from build123d import *
from build123d.topology import SkipClean

# Parameters (mm, degrees)
SKETCH1_R           = 75
SKETCH1_R_2         = 73
BOSS_EXTRUDE1_DEPTH = 25
BOSS_EXTRUDE2_START = -25
BOSS_EXTRUDE2_DEPTH = 25
SKETCH4_R           = 12
CUT_EXTRUDE2_DEPTH  = 81
BOSS_EXTRUDE3_START = 2
SKETCH5_R           = 75
SKETCH5_R_2         = 12
BOSS_EXTRUDE3_DEPTH = 2
CHAMFER1_SIZE       = 2
SKETCH6_R           = 14
SKETCH6_R_2         = 12
BOSS_EXTRUDE4_DEPTH = 50
SKETCH7_R           = 16
SKETCH7_R_2         = 14
BOSS_EXTRUDE5_DEPTH = 3
BOSS_EXTRUDE6_START = -2
SKETCH8_R           = 78
SKETCH8_R_2         = 75
BOSS_EXTRUDE6_DEPTH = 2


with BuildPart() as part:
    # Sketch1 → Boss-Extrude1 (new body)
    with BuildSketch(Plane.XY):
        Circle(SKETCH1_R)
        Circle(SKETCH1_R_2, mode=Mode.SUBTRACT)
    extrude(amount=BOSS_EXTRUDE1_DEPTH)

    # Sketch2 → Boss-Extrude2 (add)
    with BuildSketch(Plane.XY.offset(25).offset(BOSS_EXTRUDE2_START)):
        with BuildLine():
            Line((75, 81.287132565), (48, 81.287132565))
            Line((48, 81.287132565), (48, 57.628118137))
            ThreePointArc((48, 57.628118137), (67.915388536, 31.819805153), (75, 0))
            Line((75, 0), (75, 81.287132565))
        make_face()
    extrude(amount=BOSS_EXTRUDE2_DEPTH)

    # Sketch4 → Cut-Extrude2 (cut)
    with BuildSketch(Plane(origin=(0, 81.287132565, 0), x_dir=(1, 0, 0), z_dir=(0, 1, 0))):
        with Locations(Location((61.5, -12.5, 0), (0, 0, 270))):
            Circle(SKETCH4_R)
    extrude(amount=-CUT_EXTRUDE2_DEPTH, mode=Mode.SUBTRACT)

    # Sketch5 → Boss-Extrude3 (add)
    with BuildSketch(Plane(origin=(0, 0, 0), x_dir=(-1, 0, 0), z_dir=(0, 0, -1)).offset(BOSS_EXTRUDE3_START)):
        Circle(SKETCH5_R)
        Circle(SKETCH5_R_2, mode=Mode.SUBTRACT)
    extrude(amount=-BOSS_EXTRUDE3_DEPTH)

    # Chamfer1
    # the kernel refuses this chamfer: 2 mm, written as the material it takes off along each edge
    with BuildSketch(Plane(origin=(75, 81.287132565, -5.143365976), x_dir=(0.027495876610589005, -0.9996219169112968, 0), z_dir=(0, 0, 1))) as chamfer1_piece_1:
        Polygon((CHAMFER1_SIZE * 0.999621916911, -CHAMFER1_SIZE * 0.0274958766106), (-CHAMFER1_SIZE * 0.0274958766106, -CHAMFER1_SIZE * 0.999621916911), (0, 0), align=None)
    extrude(amount=35.286731952, mode=Mode.SUBTRACT)
    with BuildSketch(Plane(origin=(48, 81.287132565, -5.143365976), x_dir=(-0.02749587661058555, -0.9996219169112968, 0), z_dir=(0, 0, 1))) as chamfer1_piece_2:
        Polygon((CHAMFER1_SIZE * 0.999621916911, CHAMFER1_SIZE * 0.0274958766106), (-CHAMFER1_SIZE * 0.0274958766106, CHAMFER1_SIZE * 0.999621916911), (0, 0), align=None)
    extrude(amount=35.286731952, mode=Mode.SUBTRACT)
    with BuildSketch(Plane(origin=(80.143365976, 81.287132565, 25), x_dir=(0, -0.9996219169112968, 0.02749587661058555), z_dir=(-1, 0, 0)), Plane(origin=(80.143365976, 81.287132565, 0), x_dir=(0, 0.02749587661058908, 0.9996219169112968), z_dir=(-1, 0, 0))) as chamfer1_piece_3:
        Polygon((CHAMFER1_SIZE * 0.999621916911, -CHAMFER1_SIZE * 0.0274958766106), (-CHAMFER1_SIZE * 0.0274958766106, -CHAMFER1_SIZE * 0.999621916911), (0, 0), align=None)
    extrude(amount=37.286731952, mode=Mode.SUBTRACT)

    # Sketch6 → Boss-Extrude4 (add)
    with SkipClean():  # the faces are left unmerged after this step: merging them gives an invalid solid
        with BuildSketch(Plane.XY):
            with Locations(Location((0, 0, 0), (0, 0, 180))):
                Circle(SKETCH6_R)
            Circle(SKETCH6_R_2, mode=Mode.SUBTRACT)
        extrude(amount=BOSS_EXTRUDE4_DEPTH)
    add(part.part.scale(1), mode=Mode.REPLACE)  # the faces are merged on a copy

    # Sketch7 → Boss-Extrude5 (add)
    with BuildSketch(Plane.XY):
        with Locations(Location((0, 0, 0), (0, 0, 180))):
            Circle(SKETCH7_R)
        Circle(SKETCH7_R_2, mode=Mode.SUBTRACT)
    extrude(amount=BOSS_EXTRUDE5_DEPTH)

    # Sketch8 → Boss-Extrude6 (add)
    with SkipClean():  # the faces are left unmerged after this step: merging them gives an invalid solid
        with BuildSketch(Plane.XY.offset(25).offset(BOSS_EXTRUDE6_START)):
            Circle(SKETCH8_R)
            with Locations(Location((0, 0, 0), (0, 0, 180))):
                Circle(SKETCH8_R_2, mode=Mode.SUBTRACT)
        extrude(amount=BOSS_EXTRUDE6_DEPTH)


solid = part.part
Read the model definition and answer for the solid it produces. Units are mm, in the model's axes. A direction names the side the tool comes from. Coordinates: 2 decimals unless noted, no trailing zeros. Loops run counter-clockwise (first coordinate to the right, second up) from the corner with the lowest first, then second, coordinate; pieces in that order, holes last. Notation, with made-up numbers: (78, -11) -> (106, -11) arc R31 cw to (106, 27) -> close; hole circle Ø1 at (64, 62). An arc over 180 degrees is marked (long way). Answer in a Markdown table with one row per item.
Item 1: Straight lines are drawn through the part: line 1 along Y through (x, z) = (0, 21); line 2 along X through (y, z) = (0, -1); line 3 along Z through (x, y) = (61, 62). For each, find the intervals that lie inside material, in ascending order. Write a range as [from, to].
Returned:
| item | result |
|---|---|
| line 1 | y = [-75, -73], [-14, -12], [12, 14], [73, 75] |
| line 2 | x = [-75, -12], [12, 75] |
| line 3 | z = [0, 0.51], [24.49, 25] |
Item 2: For a pull along Y with two mould halves and no side action, classify faces 1 (the flat face through (0.07, 14.15, 3)), 2 (the flat face through (52, 81.287, 4)), 3 (the flat face through (61, 45, 23)) as released by +Y, released by -Y, zero draft, split by the parting line, or undercut.
Returned:
| item | result |
|---|---|
| face 1 | undercut |
| face 2 | released by +Y |
| face 3 | zero draft |
Item 3: A cutting plane is placed at B-B on y = 68. Determine the outline of the cut face in (x, z).
Returned:
| item | result |
|---|---|
| outline | (-38.21, 23) -> (-31.64, 23) -> (-31.64, -2) -> (31.64, -2) -> (31.64, 23) -> (38.21, 23) -> (38.21, 25) -> (26.55, 25) -> (26.55, 0) -> (-26.55, 0) -> (-26.55, 25) -> (-38.21, 25) -> close; (48, 0) -> (75, 0) -> (75, 25) -> (48, 25) -> close; hole circle Ø24 at (61.5, 12.5) |
Item 4: A cutting plane is placed at A-A on z = 12.5. Determine the outline of the cut face in (x, y), plus the area to 3 significant figures.
Returned:
| item | result |
|---|---|
| outline | circle Ø28 at (0, 0); (48, 57.63) arc R75 ccw (long way) to (75, 0) -> (75, 79.29) -> (73.5, 80.79) -> (73.5, 0.29) -> (73, 0.29) arc R73 cw (long way) to (49.5, 53.65) -> (49.5, 80.79) -> (48, 79.29) -> close; hole circle Ø24 at (0, 0) |
| area | 1,120 mm^2 |
Item 5: Each of these flat-tipped pins is pushed along its axis until it touches: P1, Ø1, axis at x = 53.5, z = 24.5, coming from the +Y side; P2, Ø24, axis at y = 70.5, z = 16.5, coming from the -X side; P3, Ø1.5, axis at x = -35.5, z = 17, coming from the -Y side. Where does it stop, or does it pass through?
Returned:
| item | result |
|---|---|
| P1 | stops at y = 80.29 |
| P2 | stops at x = -49.34 |
| P3 | stops at y = -66.46 |
Item 6: For faces 4 (the cylindrical face through (-57.93, -44.42, 12.32)), 5 (the cylindrical face through (62.177, 41.941, 23.573)), 6 (the flat face through (-75.5, 0.4, 23)), determine the directions among +Z, -Z, +X, -X, +Y, -Y from which every point of the face is accessible in a straight line to the end or side of a thin tool.
Returned:
| item | result |
|---|---|
| face 4 | +Z |
| face 5 | none |
| face 6 | -Z |
Item 7: A cutting plane is placed at C-C on x = -10. Determine the outline of the cut face in (y, z), plus the area to 3 significant figures.
Returned:
| item | result |
|---|---|
| outline | (-77.36, 23) -> (-74.33, 23) -> (-74.33, -2) -> (-6.63, -2) -> (-6.63, 50) -> (-9.8, 50) -> (-9.8, 3) -> (-12.49, 3) -> (-12.49, 0) -> (-72.31, 0) -> (-72.31, 25) -> (-77.36, 25) -> close; (6.63, -2) -> (74.33, -2) -> (74.33, 23) -> (77.36, 23) -> (77.36, 25) -> (72.31, 25) -> (72.31, 0) -> (12.49, 0) -> (12.49, 3) -> (9.8, 3) -> (9.8, 50) -> (6.63, 50) -> close |
| area | 716 mm^2 |
Item 8: A cutting plane is placed at D-D on y = -48. Determine the outline of the cut face in (x, z), plus the area to 3 significant figures.
Returned:
| item | result |
|---|---|
| outline | (-61.48, 23) -> (-57.63, 23) -> (-57.63, -2) -> (57.63, -2) -> (57.63, 23) -> (61.48, 23) -> (61.48, 25) -> (55, 25) -> (55, 0) -> (-55, 0) -> (-55, 25) -> (-61.48, 25) -> close |
| area | 377 mm^2 |
